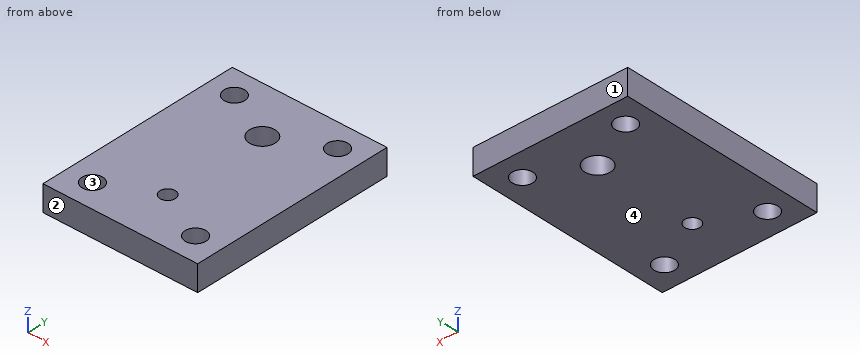
```python
from build123d import *

# Parameters (mm, degrees)
SKETCH3_W           = 38.1
SKETCH3_H           = 50.8
SKETCH3_R           = 2.5527
SKETCH3_R_2         = 3.175
SKETCH3_R_3         = 1.89865
BOSS_EXTRUDE4_DEPTH = 6.35


with BuildPart() as part:
    # Sketch3 → Boss-Extrude4 (new body)
    with BuildSketch(Plane.XY):
        with Locations((19.05, 25.4)):
            Rectangle(SKETCH3_W, SKETCH3_H)
        with Locations((6.35, 44.45)):
            Circle(SKETCH3_R, mode=Mode.SUBTRACT)
        with Locations((31.75, 44.45)):
            Circle(SKETCH3_R, mode=Mode.SUBTRACT)
        with Locations((31.75, 6.35)):
            Circle(SKETCH3_R, mode=Mode.SUBTRACT)
        with Locations((6.35, 6.35)):
            Circle(SKETCH3_R, mode=Mode.SUBTRACT)
        with Locations((19.05, 38.1)):
            Circle(SKETCH3_R_2, mode=Mode.SUBTRACT)
        with Locations((19.05, 12.7)):
            Circle(SKETCH3_R_3, mode=Mode.SUBTRACT)
    extrude(amount=BOSS_EXTRUDE4_DEPTH)


solid = part.part
```
Read the model definition and answer for the solid it produces. Units are mm, in the model's axes. Face numbers are marked on the shaded views. Give positions to 0.01 mm unless a question says otherwise; leave off trailing zeros. Write each loop counter-clockwise with the first axis right and the second up, starting at its lowest first coordinate (ties: lowest second). Pieces come first, ordered by that corner, then holes. Notation, with made-up numbers: (64.25, -39) -> (123.25, -39) arc R25 ccw to (123.25, -17) -> close; hole circle Ø5 at (27, 33.25). An arc over 180 degrees is marked (long way). Answer as a JSON object with one key per item and string values.
1) Section C-C on z = 3.25 is taken. Write down the section's boundary in (x, y) (3 decimals), then the cut area to 3 significant figures.
Findings below:
{"outline": "(0, 0) -> (38.1, 0) -> (38.1, 50.8) -> (0, 50.8) -> close; hole circle Ø5.105 at (6.35, 6.35); hole circle Ø5.105 at (6.35, 44.45); hole circle Ø6.35 at (19.05, 38.1); hole circle Ø3.797 at (19.05, 12.7); hole circle Ø5.105 at (31.75, 6.35); hole circle Ø5.105 at (31.75, 44.45)", "area": "1,810 mm^2"}
2) Straight lines are drawn through the part: probe 1 along Y at (x, z) = (6.35, 3.75); probe 2 along Y at (x, z) = (19.05, 2.5) (3 decimals); probe 3 along X at (y, z) = (44, 1.75). For each, find the intervals that lie inside material, in ascending order. Write a range as from..to.
Findings below:
{"probe 1": "y = 0..3.8, 8.9..41.9, 47..50.8", "probe 2": "y = 0..10.801, 14.599..34.925, 41.275..50.8", "probe 3": "x = 0..3.84, 8.86..29.24, 34.26..38.1"}
3) For a pull along Y with two mould halves and no side action, classify the marked faces 1, 2, 3 and 4 as pulls with the +Y half, pulls with the -Y half, needs draft (parallel to the pull), parting line crosses it, or undercut.
Findings below:
{"face 1": "pulls with the +Y half", "face 2": "pulls with the -Y half", "face 3": "undercut", "face 4": "needs draft"}
4) Section D-D on y = 6.35 is taken. Write down the section's boundary in (x, z).
Findings below:
{"outline": "(0, 0) -> (3.8, 0) -> (3.8, 6.35) -> (0, 6.35) -> close; (8.9, 0) -> (29.2, 0) -> (29.2, 6.35) -> (8.9, 6.35) -> close; (34.3, 0) -> (38.1, 0) -> (38.1, 6.35) -> (34.3, 6.35) -> close"}
5) Section A-A on y = 38.1 is taken. Write down the section's boundary in (x, z) (3 decimals), then the cut area to 3 significant figures.
Findings below:
{"outline": "(0, 0) -> (15.875, 0) -> (15.875, 6.35) -> (0, 6.35) -> close; (22.225, 0) -> (38.1, 0) -> (38.1, 6.35) -> (22.225, 6.35) -> close", "area": "202 mm^2"}
6) Section B-B on x = 31.75 is taken. Write down the section's boundary in (y, z), then the cut area to 3 significant figures.
Findings below:
{"outline": "(0, 0) -> (3.8, 0) -> (3.8, 6.35) -> (0, 6.35) -> close; (8.9, 0) -> (41.9, 0) -> (41.9, 6.35) -> (8.9, 6.35) -> close; (47, 0) -> (50.8, 0) -> (50.8, 6.35) -> (47, 6.35) -> close", "area": "258 mm^2"}
